Can you work these out from the model? Positions are in its coordinate system, mm. A direction names the side the tool comes from. Round coordinates to 2 decimals unless told otherwise and drop trailing zeros. Write each loop counter-clockwise with the first axis right and the second up, starting at its lowest first coordinate (ties: lowest second). Pieces come first, ordered by that corner, then holes. Notation, with made-up numbers: (-19, 31.5) - (-8, 31.5) arc R28 cw to (-8, 62.5) - close; hole circle Ø3 at (59.25, 81.5). An arc over 180 degrees is marked (long way). One line per item, written item: value. Start each with the question number.
(1) On a 3-axis mill with a long thin cutter (end or side, diameter ignored), from which of +Z, -Z, +X, -X, +Y, -Y can I reach the whole of each face in a straight line? I mean faces 1 (the face through (0, -3.835, 0)), 2 (the face through (19.05, -10, 6)), 3 (the face through (-27, 13, -3.175)). Say none if no direction works.
(2) If I drill on L1, parallel to Z at x = 5.08, y = -6.25; L2, parallel to X at y = -2, z = -6.5; L3, parallel to X at y = 9.5, z = -3.25, over which ranges is the centre line in solid material (lowest first)? Write a range as from..to.
(3) I want a section at D-D on y = 12. List the corners of the cut face in (x, z) for me (3 decimals), plus the area to 3 significant figures.
(4) I'm going to push flat-ended pins straight in: pin 1 Ø12 at (x, z) = (-11, 3) entering from +Y; pin 2 Ø2.5 at (y, z) = (14, -1) entering from +X; pin 3 Ø3.5 at (x, y) = (24.13, 9.525) entering from +Z; pin 4 Ø3 at (x, y) = (-26.67, 4.445) entering from +Z. Where does each tip first touch, or does it pass through?
(5) I want a section at A-A on y = -6. List the corners of the cut face in (x, z) for me.
(6) I want a section at C-C on x = -10.16. List the corners of the cut face in (y, z) for me (3 decimals).
(7) I want a section at B-B on z = -7.5. List the corners of the cut face in (x, y) for me (3 decimals), plus the area to 3 significant figures.
(8) Thinking about a two-plate mould opening in X: for faces 4 (the face through (20.32, 6, -6)), 5 (the face through (-28, 9.525, -2)), 6 (the face through (24.13, 13, -2)), 7 (the face through (-24.13, 13, -2)), which applies, +X half, -X half, draft (parallel to the pull), parting line (faces both ways), or undercut?
from build123d import *

# Parameters (mm, degrees)
SKETCH1_W                 = 60.96
SKETCH1_H                 = 31.75
BOSS_EXTRUDE1_DEPTH       = 12.7
CUT_EXTRUDE2_REACH        = 27.4
SKETCH4_W                 = 40.64
SKETCH4_H                 = 19.7104
SKETCH5_W                 = 11.43
SKETCH5_H                 = 31.75
CUT_EXTRUDE3_DEPTH        = 12.7
SKETCH6_W                 = 6.35
SKETCH6_H                 = 6.35
CUT_EXTRUDE4_DEPTH        = 3.175
SKETCH7_R                 = 1.5875
CUT_EXTRUDE5_DEPTH        = 6.35
F_8_32_TAPPED_HOLE1_D     = 3.4544
F_8_32_TAPPED_HOLE1_DEPTH = 12.701
CUT_EXTRUDE6_REACH        = 14.04
SKETCH10_R                = 2.2352


with BuildPart() as part:
    # Sketch1 → Boss-Extrude1 (new body, symmetric)
    with BuildSketch(Plane.XY):
        Rectangle(SKETCH1_W, SKETCH1_H)
    extrude(amount=BOSS_EXTRUDE1_DEPTH, both=True)

    # Sketch4 → Cut-Extrude2 (cut, up to next)
    with BuildSketch(Plane.XY.offset(12.7), mode=Mode.PRIVATE) as cut_extrude2_sk1:
        with Locations((0, 6.0198)):
            Rectangle(SKETCH4_W, SKETCH4_H)
    cut_extrude2_tool1 = extrude(cut_extrude2_sk1.sketch, amount=-CUT_EXTRUDE2_REACH, mode=Mode.PRIVATE) & part.part
    add(cut_extrude2_tool1.solids().sort_by_distance((0, 6.0198, 12.7))[0], mode=Mode.SUBTRACT)

    # Sketch5 → Cut-Extrude3 (cut)
    with BuildSketch(Plane.XY.offset(12.7)):
        with Locations((24.765, 0)):
            Rectangle(SKETCH5_W, SKETCH5_H)
    cut_extrude3 = extrude(amount=-CUT_EXTRUDE3_DEPTH, mode=Mode.SUBTRACT)

    # Mirror2: Cut-Extrude3 across plane
    add(cut_extrude3.mirror(Plane(origin=(0, 0, 0), x_dir=(0, 0, 1), z_dir=(1, 0, 0))), mode=Mode.SUBTRACT)

    # Sketch6 → Cut-Extrude4 (cut)
    with BuildSketch(Plane.XY):
        with Locations((27.305, 12.7)):
            Rectangle(SKETCH6_W, SKETCH6_H)
    cut_extrude4 = extrude(amount=-CUT_EXTRUDE4_DEPTH, mode=Mode.SUBTRACT)

    # Sketch7 → Cut-Extrude5 (cut)
    with BuildSketch(Plane.XY):
        with Locations((24.13, 9.525)):
            Circle(SKETCH7_R)
    cut_extrude5 = extrude(amount=-CUT_EXTRUDE5_DEPTH, mode=Mode.SUBTRACT)

    # #8-32 Tapped Hole1
    with Locations(Plane.XY):
        with Locations((26.67, 4.445)):
            f_8_32_tapped_hole1 = Hole(F_8_32_TAPPED_HOLE1_D / 2, depth=F_8_32_TAPPED_HOLE1_DEPTH)

    # Sketch10 → Cut-Extrude6 (cut, up to next)
    with BuildSketch(Plane(origin=(0, -3.8354, 0), x_dir=(1, 0, 0), z_dir=(0, 1, 0)), mode=Mode.PRIVATE) as cut_extrude6_sk1:
        with Locations((5.08, 8.89)):
            Circle(SKETCH10_R)
    cut_extrude6_tool1 = extrude(cut_extrude6_sk1.sketch, amount=-CUT_EXTRUDE6_REACH, mode=Mode.PRIVATE) & part.part
    add(cut_extrude6_tool1.solids().sort_by_distance((5.08, -3.8354, -8.89))[0], mode=Mode.SUBTRACT)
    # Sketch10 → Cut-Extrude6 (cut, up to next)
    with BuildSketch(Plane(origin=(0, -3.8354, 0), x_dir=(1, 0, 0), z_dir=(0, 1, 0)), mode=Mode.PRIVATE) as cut_extrude6_sk2:
        with Locations((5.08, -8.89)):
            Circle(SKETCH10_R)
    cut_extrude6_tool2 = extrude(cut_extrude6_sk2.sketch, amount=-CUT_EXTRUDE6_REACH, mode=Mode.PRIVATE) & part.part
    add(cut_extrude6_tool2.solids().sort_by_distance((5.08, -3.8354, 8.89))[0], mode=Mode.SUBTRACT)
    # Sketch10 → Cut-Extrude6 (cut, up to next)
    with BuildSketch(Plane(origin=(0, -3.8354, 0), x_dir=(1, 0, 0), z_dir=(0, 1, 0)), mode=Mode.PRIVATE) as cut_extrude6_sk3:
        with Locations((-10.16, 0)):
            Circle(SKETCH10_R)
    cut_extrude6_tool3 = extrude(cut_extrude6_sk3.sketch, amount=-CUT_EXTRUDE6_REACH, mode=Mode.PRIVATE) & part.part
    add(cut_extrude6_tool3.solids().sort_by_distance((-10.16, -3.8354, 0))[0], mode=Mode.SUBTRACT)

    # Mirror3: Cut-Extrude4, Cut-Extrude5, #8-32 Tapped Hole1 across plane
    add(cut_extrude4.mirror(Plane(origin=(0, 0, 0), x_dir=(0, 0, 1), z_dir=(1, 0, 0))), mode=Mode.SUBTRACT)
    add(cut_extrude5.mirror(Plane(origin=(0, 0, 0), x_dir=(0, 0, 1), z_dir=(1, 0, 0))), mode=Mode.SUBTRACT)
    add(f_8_32_tapped_hole1.mirror(Plane(origin=(0, 0, 0), x_dir=(0, 0, 1), z_dir=(1, 0, 0))), mode=Mode.SUBTRACT)


solid = part.part
Established:
1. face 1: +Z, -Z, +Y
1. face 2: +Z, +X, +Y, -Y
1. face 3: +Z, -X, +Y
2. L1: -12.7..-11.13, -6.65..6.65, 11.13..12.7
2. L2: -30.48..-20.32, 20.32..30.48
2. L3: -30.48..-25.72, -22.54..-20.32, 20.32..22.54, 25.72..30.48
3. outline: (-30.48, -12.7) - (-20.32, -12.7) - (-20.32, 0) - (-24.13, 0) - (-24.13, -3.175) - (-30.48, -3.175) - close; (20.32, -12.7) - (30.48, -12.7) - (30.48, -3.175) - (24.13, -3.175) - (24.13, 0) - (20.32, 0) - close
3. area: 218 mm2
4. pin 1: y = -3.84
4. pin 2: x = 24.13
4. pin 3: z = 0
4. pin 4: through
5. outline: (-30.48, -12.7) - (30.48, -12.7) - (30.48, 0) - (19.05, 0) - (19.05, 12.7) - (-19.05, 12.7) - (-19.05, 0) - (-30.48, 0) - close; hole circle Ø4.47 at (-10.16, 0); hole circle Ø4.47 at (5.08, -8.89); hole circle Ø4.47 at (5.08, 8.89)
6. outline: (-15.875, -12.7) - (-3.835, -12.7) - (-3.835, -2.235) - (-15.875, -2.235) - close; (-15.875, 2.235) - (-3.835, 2.235) - (-3.835, 12.7) - (-15.875, 12.7) - close
7. outline: (-30.48, -15.875) - (3.33, -15.875) - (3.33, -3.835) - (-20.32, -3.835) - (-20.32, 15.875) - (-30.48, 15.875) - close; (6.83, -15.875) - (30.48, -15.875) - (30.48, 15.875) - (20.32, 15.875) - (20.32, -3.835) - (6.83, -3.835) - close; hole circle Ø3.454 at (-26.67, 4.445); hole circle Ø3.454 at (26.67, 4.445)
7. area: 1,070 mm2
8. face 4: undercut
8. face 5: draft
8. face 6: +X half
8. face 7: -X half
